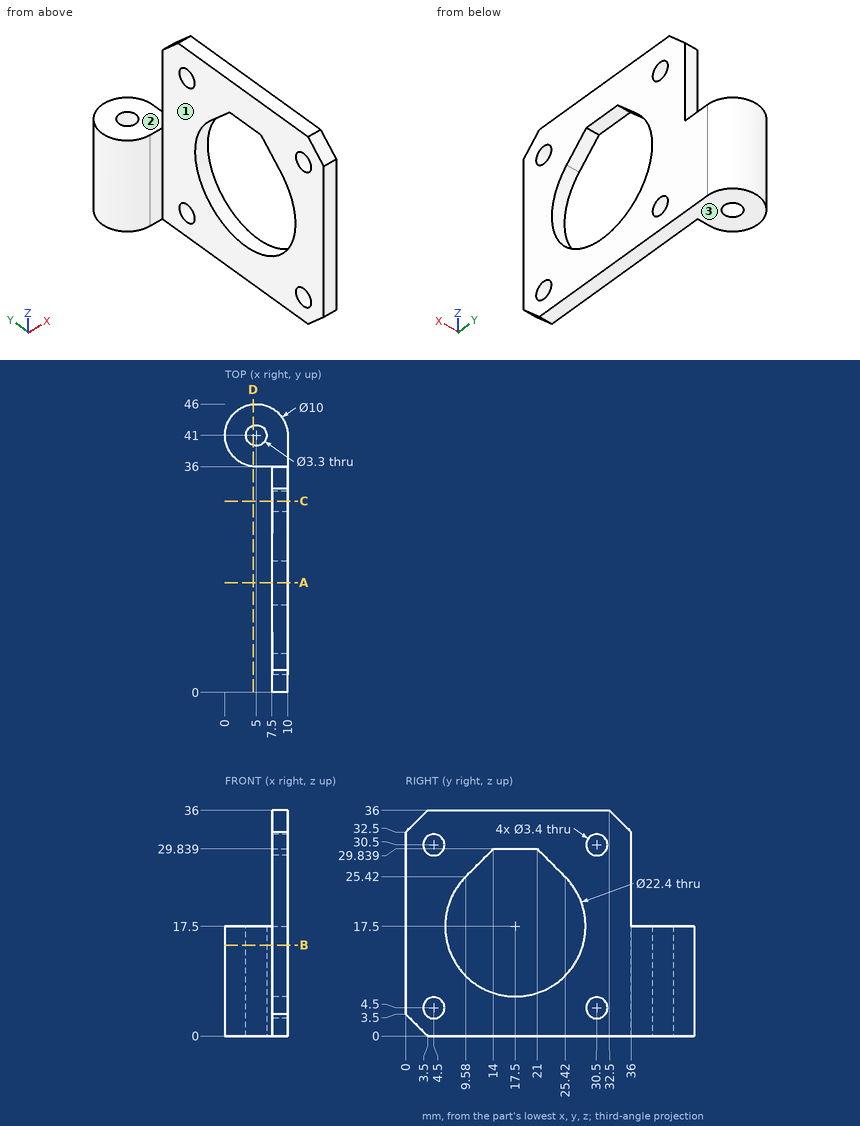
Could you check a few things on this drawing? It's one solid part, dimensions in mm from its lowest x, y, z. A direction names the side the tool comes from. Give positions to 0.01 mm unless a question says otherwise; leave off trailing zeros. Order: outer loops, then holes, each group sorted by start corner. A loop starts at its lowest first (then second) coordinate and runs counter-clockwise, first axis right, second up. Notation, with made-up numbers: M 47.25,-10 L 56.25,-10 A31 cw 56.25,22 Z; hole C 40,31 d10. An arc over 180 degrees is marked long. Use one line per item in the form item = value. Start each with the question number.
Item 1: If we section it at D-D (x = 4.5): Write out the boundary of the cut face in (y, z) (1 decimal).
Item 2: For the marked faces 1, 2 and 3, which set-ups out of +Z, -Z, +X, -X, +Y, -Y let a thin tool reach every point of the face, with its end or its side?
Item 3: If we section it at B-B (z = 14.5): Write out the boundary of the cut face in (x, y), then the cut area to 3 significant figures.
Item 4: If we section it at A-A (y = 17.5): Write out the boundary of the cut face in (x, z).
Item 5: Will these pins go through, and if not, where does the flat tip stop? pin 1 Ø18 at (y, z) = (19.5, 26.5) entering from -X; pin 2 Ø1.3 at (x, z) = (8.5, 27.5) entering from +Y; pin 3 Ø10 at (y, z) = (35.5, 10.5) entering from -X (1 decimal).
Item 6: If I drill on line 1 along Z through (x, y) = (8.9, 4.5); line 2 along Z through (x, y) = (8.75, 17.5); line 3 along Z through (x, y) = (8.25, 5.5) (1 decimal), over which ranges is the centre line in solid material (lowest first)?
Item 7: If we section it at C-C (y = 30.5): Write out the boundary of the cut face in (x, z).
Outcome:
q1.outline = M 36,0 L 39.4,0 L 39.4,17.5 L 36,17.5 Z; M 42.6,0 L 46,0 L 46,17.5 L 42.6,17.5 Z
q2.face_1 = +Z, -Z, -X, -Y
q2.face_2 = +Z, +X, -X, +Y
q2.face_3 = -Z, +X, -X, +Y, -Y
q3.outline = M 5,36 L 7.5,36 L 7.5,28.29 L 10,28.29 L 10,41 A5 ccw long Z; M 7.5,0 L 10,0 L 10,6.71 L 7.5,6.71 Z; hole C 5,41 d3.3
q3.area = 111 mm2
q4.outline = M 7.5,0 L 10,0 L 10,6.3 L 7.5,6.3 Z; M 7.5,29.84 L 10,29.84 L 10,36 L 7.5,36 Z
q5.pin_1 = 7.5
q5.pin_2 = 36
q5.pin_3 = 0
q6.line_1 = 0 to 2.8, 6.2 to 28.8, 32.2 to 36
q6.line_2 = 0 to 6.3, 29.84 to 36
q6.line_3 = 0 to 3.1, 5.9 to 29.1, 31.9 to 36
q7.outline = M 7.5,0 L 10,0 L 10,2.8 L 7.5,2.8 Z; M 7.5,6.2 L 10,6.2 L 10,28.8 L 7.5,28.8 Z; M 7.5,32.2 L 10,32.2 L 10,36 L 7.5,36 Z
